```python
from build123d import *

# Parameters (mm, degrees)
F1_DEPTH      = 16
F3_D          = 18
F5_D          = 18
F6_ANGLE      = 45
F8_START      = -100
F8_DEPTH      = 160
F9_DEPTH      = 100
F9_DEPTH_BACK = 100
F10_T1_DEPTH  = 32
F10_T3_DEPTH  = 32
F10_T5_DEPTH  = 360
F10_T7_DEPTH  = 160
F10_T9_DEPTH  = 157
F10_T11_DEPTH = 157
F10_T13_DEPTH = 485
F10_T15_DEPTH = 285
F11_SIZE      = 3
F13_D         = 10


# Not quite as in the source:
# - a fillet or chamfer that OpenCascade refuses, or shapes differently, is made with other operations: its cross-section is extruded or revolved along the edge and cut away or added


with BuildPart() as f1:
    # F0 (on Front) → F1 (new body, symmetric)
    with BuildSketch(Plane.XZ):
        Polygon((-95, 16), (-105, 16), (-105, -16), (-105, -174), (105, -174), (105, -16), (105, 16), (95, 16), (95, -16), (95, -154), (-95, -154), (-95, -16), align=None)
        Polygon((-105, 174), (-105, 16), (-95, 16), (-95, 154), (95, 154), (95, 16), (105, 16), (105, 174), align=None)
    extrude(amount=F1_DEPTH, both=True)

    # F3 (through all)
    with Locations(Plane.YZ.offset(105)):
        with Locations((0, 0)):
            Hole(F3_D / 2)

    # F5 (through all)
    with Locations(Plane.XY.offset(174)):
        with Locations((0, 0)):
            Hole(F5_D / 2)


with BuildPart() as f1_1:
    # F6: moved
    add(f1.part.rotate(Axis((0, 0, 16), (1, 0, 0)), F6_ANGLE))

    # F7 (on Top) → F8 (join)
    with BuildSketch(Plane.XY.offset(F8_START)):
        Polygon((0, 1010), (-105, 1010), (-105, -220), (-95, -220), (-95, 1000), (0, 1000), (95, 1000), (95, -220), (105, -220), (105, 1010), align=None)
        Polygon((-95, -220), (-105, -220), (-105, -460), (0, -460), (105, -460), (105, -220), (95, -220), (95, -450), (0, -450), (-95, -450), align=None)
    extrude(amount=-F8_DEPTH)

    # F7 (on Top) → F9 (join, two sides)
    with BuildSketch(Plane.XY) as f9_sk:
        Polygon((-95, -220), (-105, -220), (-105, -460), (0, -460), (105, -460), (105, -220), (95, -220), (95, -450), (0, -450), (-95, -450), align=None)
    extrude(amount=F9_DEPTH)
    extrude(f9_sk.sketch, amount=-F9_DEPTH_BACK)

    # F10: fillet of radius 25 on 14 edges, made by hand

    # F10_s2 → F10_t1 (join)
    with BuildSketch(Plane(origin=(0, -3.313708499, -3.313708499), x_dir=(1, 0, 0), z_dir=(0, 0.7071067812, 0.7071067812))):
        with BuildLine():
            ThreePointArc((-95, 133.686291501), (-87.6776695297, 151.3639610307), (-70, 158.686291501))
            Line((-70, 158.686291501), (-95, 158.686291501))
            Line((-95, 158.686291501), (-95, 133.686291501))
        make_face()
    extrude(amount=F10_T1_DEPTH)

    # F10_s4 → F10_t3 (join)
    with BuildSketch(Plane(origin=(0, 19.313708499, 19.313708499), x_dir=(1, 0, 0), z_dir=(0, -0.7071067812, -0.7071067812))):
        with BuildLine():
            ThreePointArc((70, -158.686291501), (87.6776695297, -151.3639610307), (95, -133.686291501))
            Line((95, -133.686291501), (95, -158.686291501))
            Line((95, -158.686291501), (70, -158.686291501))
        make_face()
        with BuildLine():
            ThreePointArc((95, 124.313708499), (87.6776695297, 141.9913780286), (70, 149.313708499))
            Line((70, 149.313708499), (95, 149.313708499))
            Line((95, 149.313708499), (95, 124.313708499))
        make_face()
        with BuildLine():
            ThreePointArc((-95, 124.313708499), (-87.6776695297, 141.9913780286), (-70, 149.313708499))
            Line((-70, 149.313708499), (-95, 149.313708499))
            Line((-95, 149.313708499), (-95, 124.313708499))
        make_face()
    extrude(amount=F10_T3_DEPTH)

    # F10_s6 → F10_t5 (join)
    with BuildSketch(Plane.XY.offset(-260)):
        with BuildLine():
            ThreePointArc((-95, -425), (-87.6776695297, -442.6776695297), (-70, -450))
            Line((-70, -450), (-95, -450))
            Line((-95, -450), (-95, -425))
        make_face()
        with BuildLine():
            ThreePointArc((95, -425), (87.6776695297, -442.6776695297), (70, -450))
            Line((70, -450), (95, -450))
            Line((95, -450), (95, -425))
        make_face()
    extrude(amount=F10_T5_DEPTH)

    # F10_s8 → F10_t7 (join)
    with BuildSketch(Plane.XY.offset(-260)):
        with BuildLine():
            ThreePointArc((95, 975), (87.6776695297, 992.6776695297), (70, 1000))
            Line((70, 1000), (95, 1000))
            Line((95, 1000), (95, 975))
        make_face()
        with BuildLine():
            ThreePointArc((-95, 975), (-87.6776695297, 992.6776695297), (-70, 1000))
            Line((-70, 1000), (-95, 1000))
            Line((-95, 1000), (-95, 975))
        make_face()
    extrude(amount=F10_T7_DEPTH)

    # F10_s10 → F10_t9 (cut)
    with BuildSketch(Plane(origin=(0, 63.5078823231, 63.5078823231), x_dir=(1, 0, 0), z_dir=(0, -0.7071067812, -0.7071067812))):
        with BuildLine():
            ThreePointArc((105, 144.313708499), (97.6776695297, 161.9913780286), (80, 169.313708499))
            Line((80, 169.313708499), (105, 169.313708499))
            Line((105, 169.313708499), (105, 144.313708499))
        make_face()
    extrude(amount=F10_T9_DEPTH, mode=Mode.SUBTRACT)

    # F10_s12 → F10_t11 (cut)
    with BuildSketch(Plane(origin=(0, -47.5078823231, -47.5078823231), x_dir=(1, 0, 0), z_dir=(0, 0.7071067812, 0.7071067812))):
        with BuildLine():
            ThreePointArc((-105, -144.313708499), (-97.6776695297, -161.9913780286), (-80, -169.313708499))
            Line((-80, -169.313708499), (-105, -169.313708499))
            Line((-105, -169.313708499), (-105, -144.313708499))
        make_face()
    extrude(amount=F10_T11_DEPTH, mode=Mode.SUBTRACT)

    # F10_s14 → F10_t13 (cut)
    with BuildSketch(Plane.XY.offset(-322.5)):
        with BuildLine():
            ThreePointArc((-105, -435), (-97.6776695297, -452.6776695297), (-80, -460))
            Line((-80, -460), (-105, -460))
            Line((-105, -460), (-105, -435))
        make_face()
        with BuildLine():
            ThreePointArc((105, -435), (97.6776695297, -452.6776695297), (80, -460))
            Line((80, -460), (105, -460))
            Line((105, -460), (105, -435))
        make_face()
    extrude(amount=F10_T13_DEPTH, mode=Mode.SUBTRACT)

    # F10_s16 → F10_t15 (cut)
    with BuildSketch(Plane.XY.offset(-322.5)):
        with BuildLine():
            ThreePointArc((105, 985), (97.6776695297, 1002.6776695297), (80, 1010))
            Line((80, 1010), (105, 1010))
            Line((105, 1010), (105, 985))
        make_face()
        with BuildLine():
            ThreePointArc((-105, 985), (-97.6776695297, 1002.6776695297), (-80, 1010))
            Line((-80, 1010), (-105, 1010))
            Line((-105, 1010), (-105, 985))
        make_face()
    extrude(amount=F10_T15_DEPTH, mode=Mode.SUBTRACT)

    # F11
    f11_edges = [f1_1.edges().sort_by_distance(p)[0] for p in [
        (97.67767, -95.231493, 133.85891),
        (97.67767, -117.85891, 111.231493),
    ]]
    chamfer(f11_edges, length=F11_SIZE)

    # F13 (through all)
    with Locations(Plane.YZ.offset(105)):
        with Locations((-314.7462682585, 29.8209178701), (-261.1231572401, -15.1742148079), (-338.2576704025, -107.0995479822), (-391.8807814209, -62.1044153042)):
            Hole(F13_D / 2)


solid = f1_1.part
```
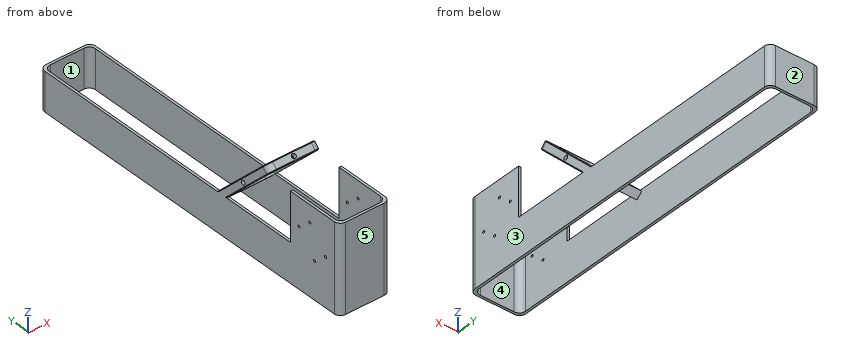
Geometry check sheet. Reference: the model listing, model coordinates, mm. Face numbers are marked on the shaded views. A direction names the side the tool comes from. Coordinates: 2 decimals unless noted, no trailing zeros. Loops run counter-clockwise (first coordinate to the right, second up) from the corner with the lowest first, then second, coordinate; pieces in that order, holes last.
Item 1: Sectioned sample at B-B, the plane x = -25.5. Record the boundary of the cut face in (y, z), then the cut area to 3 significant figures.
Item 2: Sectioned sample at D-D, the plane y = -37. Record the boundary of the cut face in (x, z).
Item 3: Go/stop test with flat-tipped pins: pin 1 Ø8 at (y, z) = (-314.75, 29.82) entering from +X; pin 2 Ø5 at (x, y) = (98.5, -22) entering from +Z. Record where each tip stops, or that it passes through.
Item 4: Access from +Z, -Z, +X, -X, +Y, -Y to the whole of each face (thin tool, end or side, straight path). Record for the marked faces 1 and 2.
Item 5: Release check for a two-part mould opening along Y. For the marked faces 3, 4 and 5 record: released by +Y, released by -Y, zero draft, split by the parting line, or undercut.
Item 6: Sectioned sample at C-C, the plane z = 69. Record the boundary of the cut face in (x, y), then the cut area to 3 significant figures.
Item 7: Thickness scan on line 1 (Y direction, x = -59.5, z = -194.5); line 2 (X direction, y = 364, z = -233); line 3 (Y direction, x = -26.5, z = 10.5). Record the ranges inside material, lowest first.
Item 8: Sectioned sample at A-A, the plane y = 826.5. Record the boundary of the cut face in (x, z).
Check result:
1. outline: (-460, -260) - (-450, -260) - (-450, 100) - (-460, 100) - close; (-120.92, 114.29) - (-108.89, 102.27) - (-86.27, 124.89) - (-98.29, 136.92) - (-102.53, 136.92) - (-120.92, 118.53) - close; (108.89, -115.52) - (123.04, -129.66) - (145.66, -107.04) - (131.52, -92.89) - close; (1000, -260) - (1010, -260) - (1010, -100) - (1000, -100) - close
1. area: 6,470 mm2
2. outline: (-105, -260) - (-95, -260) - (-95, -100) - (-105, -100) - close; (-105, 34.62) - (-102, 30.37) - (-95, 30.37) - (-95, 75.63) - (-102, 75.63) - (-105, 71.38) - close; (95, -260) - (105, -260) - (105, -100) - (95, -100) - close; (95, 30.37) - (102, 30.37) - (105, 34.62) - (105, 71.38) - (102, 75.63) - (95, 75.63) - close
3. pin 1: passes through
3. pin 2: stops at z = 63.13
4. face 1: +Z, -Z
4. face 2: +Z, -Z, +X, -X, +Y
5. face 3: zero draft
5. face 4: undercut
5. face 5: released by -Y
6. outline: (-105, -435) arc R25 ccw to (-80, -460) - (80, -460) arc R25 ccw to (105, -435) - (105, -220) - (95, -220) - (95, -425) arc R25 cw to (70, -450) - (-70, -450) arc R25 cw to (-95, -425) - (-95, -220) - (-105, -220) - close; (-105, -71.38) - (-102, -75.63) - (-95, -75.63) - (-95, -30.37) - (-102, -30.37) - (-105, -34.62) - close; (95, -75.63) - (102, -75.63) - (105, -71.38) - (105, -34.62) - (102, -30.37) - (95, -30.37) - close
6. area: 7,580 mm2
7. line 1: y = -460 to -450, 1000 to 1010
7. line 2: x = -105 to -95, 95 to 105
7. line 3: y = -460 to -450
8. outline: (-105, -260) - (-95, -260) - (-95, -100) - (-105, -100) - close; (95, -260) - (105, -260) - (105, -100) - (95, -100) - close
